from build123d import *

# Parameters (mm, degrees)
SKETCH1_W                = 22
SKETCH1_H                = 22
SKETCH1_R                = 1.65
BOSS_EXTRUDE1_DEPTH      = 5
SKETCH2_W                = 5
SKETCH2_H                = 22
BOSS_EXTRUDE2_DEPTH      = 10
SKETCH3_W                = 7
SKETCH3_H                = 10
CUT_EXTRUDE1_DEPTH       = 0.1
FILLET1_R                = 10
SKETCH5_W                = 35
SKETCH5_H                = 15
SKETCH5_R                = 1.75
CHANGE_THIS_SKETCH_DEPTH = 5
FILLET2_R                = 3


with BuildPart() as part:
    # Sketch1 → Boss-Extrude1 (new body)
    with BuildSketch(Plane(origin=(0, 0, 0), x_dir=(1, 0, 0), z_dir=(0, 1, 0))):
        with Locations((11, 11)):
            Rectangle(SKETCH1_W, SKETCH1_H)
        with Locations(Location((13.5, 11, 0), (0, 0, 270))):
            Circle(SKETCH1_R, mode=Mode.SUBTRACT)
        with Locations(Location((3.5, 3.5, 0), (0, 0, 270))):
            Circle(SKETCH1_R, mode=Mode.SUBTRACT)
        with Locations(Location((3.5, 18.5, 0), (0, 0, 90))):
            Circle(SKETCH1_R, mode=Mode.SUBTRACT)
    extrude(amount=BOSS_EXTRUDE1_DEPTH)

    # Sketch2 → Boss-Extrude2 (add)
    with BuildSketch(Plane(origin=(0, 5, 0), x_dir=(1, 0, 0), z_dir=(0, 1, 0))):
        with Locations((19.5, 11)):
            Rectangle(SKETCH2_W, SKETCH2_H)
    extrude(amount=BOSS_EXTRUDE2_DEPTH)

    # Sketch3 → Cut-Extrude1 (cut)
    with BuildSketch(Plane.ZY.offset(-17)):
        with Locations((-11, 10)):
            Rectangle(SKETCH3_W, SKETCH3_H)
    extrude(amount=-CUT_EXTRUDE1_DEPTH, mode=Mode.SUBTRACT)

    # Fillet1
    fillet1_edges = [part.edges().sort_by_distance(p)[0] for p in [
        (17, 5, -18.25),
        (17, 5, -3.75),
    ]]
    fillet(fillet1_edges, radius=FILLET1_R - 0.0001)  # a hair under: the kernel refuses the full size

    # Sketch5 → CHANGE THIS SKETCH (add)
    with BuildSketch(Plane(origin=(22, 0, 0), x_dir=(0, 0, -1), z_dir=(1, 0, 0))):
        with Locations((11, 22.5)):
            Rectangle(SKETCH5_W, SKETCH5_H)
        with Locations((23.5, 22.5)):
            Circle(SKETCH5_R, mode=Mode.SUBTRACT)
        with Locations((-1.5, 22.5)):
            Circle(SKETCH5_R, mode=Mode.SUBTRACT)
    extrude(amount=-CHANGE_THIS_SKETCH_DEPTH)

    # Fillet2
    fillet2_edges = [part.edges().sort_by_distance(p)[0] for p in [
        (19.5, 15, -22),
        (19.5, 15, 0),
        (0, 2.5, -22),
        (19.5, 15, 6.5),
        (19.5, 30, 6.5),
        (19.5, 30, -28.5),
        (19.5, 15, -28.5),
        (0, 2.5, 0),
    ]]
    fillet(fillet2_edges, radius=FILLET2_R)


solid = part.part
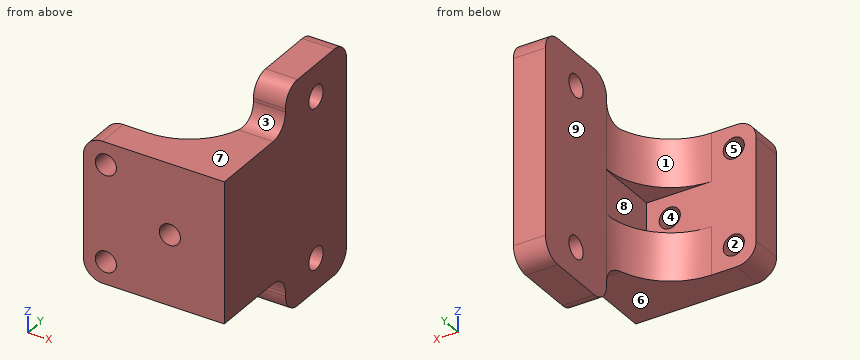
Model file for the job. Use its own axes, mm. Face numbers are marked on the shaded views. A direction names the side the tool comes from. Coordinates: 2 decimals unless noted, no trailing zeros. Order: outer loops, then holes, each group sorted by start corner. A loop starts at its lowest first (then second) coordinate and runs counter-clockwise, first axis right, second up. Notation, with made-up numbers: (8.25, 83.25) -> (23.25, 83.25) arc R15 ccw to (23.25, 106.25) -> close; hole circle Ø11 at (72.25, 25.25). An arc over 180 degrees is marked (long way). Return JSON: item names as keys, results as strings. Group by question number.
Item 1: Saw through at D-D on x = 13.5. Write the cut outline in (y, z).
Item 2: Saw through at B-B on z = -18.5. Write the cut outline in (x, y), then the cut area to 3 significant figures.
Item 3: Wall check: line 1 along X through (y, z) = (2.6, -18.5); line 2 along Z through (x, y) = (12, 5.25); line 3 along Z through (x, y) = (19.25, 24). Give the ranges that are in metal, low to high. Write a range as [from, to].
Item 4: Saw through at A-A on y = 4. Write the cut outline in (x, z).
Item 5: Saw through at C-C on x = 18.75. Write the cut outline in (y, z).
Item 6: Pull direction X, two halves, no side cores. Call the marked faces 1, 2, 3 and 4: pulls with the +X half, pulls with the -X half, needs draft (parallel to the pull), parting line crosses it, or undercut.
Item 7: Flat gauge pins, fed straight in: P1, Ø2, axis at y = 11.5, z = -11.5, coming from the -X side; P2, Ø10, axis at x = 11, z = -5, coming from the -Y side; P3, Ø8.5, axis at x = 6, z = -10.5, coming from the +Y side; P4, Ø16.5, axis at y = 19, z = -3.5, coming from the -X side. Where does each tip first touch, or does it go through?
Item 8: Tool access for the marked faces 5, 6, 7, 8 and 9: list every direction of +Z, -Z, +X, -X, +Y, -Y with a clear straight run to the whole face (end or side of a thin tool).
Values found:
{
 "1": {"outline": "(0, -22) -> (7.4, -22) -> (7.4, -14.5) -> (5, -14.5) -> (5, -12.65) -> (0, -12.65) -> close; (0, -9.35) -> (5, -9.35) -> (5, -7.5) -> (7.4, -7.5) -> (7.4, 0) -> (0, 0) -> close"},
 "2": {"outline": "(0, 0) -> (1.85, 0) -> (1.85, 5) -> (0, 5) -> close; (5.15, 0) -> (22, 0) -> (22, 30) -> (17, 30) -> (17, 15) arc R10 cw to (7, 5) -> (5.15, 5) -> close", "area": "240 mm2"},
 "3": {"line 1": "x = [0, 1.85], [5.15, 22]", "line 2": "z = [-22, -14.5], [-7.5, 0]", "line 3": "z = [-28.5, -24.4], [-22.6, 0.6], [2.4, 6.5]"},
 "4": {"outline": "(0, -19) arc R3 ccw to (3, -22) -> (22, -22) -> (22, 0) -> (3, 0) arc R3 ccw to (0, -3) -> close; hole circle Ø3.3 at (3.5, -18.5); hole circle Ø3.3 at (3.5, -3.5); hole circle Ø3.3 at (13.5, -11)"},
 "5": {"outline": "(0, -22) -> (12, -22) arc R3 cw to (15, -25) -> (15, -25.5) arc R3 ccw to (18, -28.5) -> (27, -28.5) arc R3 ccw to (30, -25.5) -> (30, 3.5) arc R3 ccw to (27, 6.5) -> (18, 6.5) arc R3 ccw to (15, 3.5) -> (15, 3) arc R3 cw to (12, 0) -> (0, 0) -> close; hole circle Ø3.5 at (22.5, -23.5); hole circle Ø3.5 at (22.5, 1.5)"},
 "6": {"face 1": "pulls with the -X half", "face 2": "undercut", "face 3": "needs draft", "face 4": "undercut"},
 "7": {"P1": "stops at x = 17.1", "P2": "stops at y = 0", "P3": "stops at y = 5.2", "P4": "stops at x = 16.05"},
 "8": {"face 5": "+Y, -Y", "face 6": "-Z, +X, -X, -Y", "face 7": "+Z, +X, -X, -Y", "face 8": "-X", "face 9": "+Z, -Z, -X, +Y"}
}
